Here's how the part is built. I have some questions about the finished solid (model axes, mm). Round coordinates to 2 decimals unless told otherwise and drop trailing zeros. Loops run counter-clockwise (first coordinate to the right, second up) from the corner with the lowest first, then second, coordinate; pieces in that order, holes last. Notation, with made-up numbers: M 81.5,-33 L 113.5,-33 A7 cw 113.5,-28 Z; hole C 42,62 d4. An arc over 180 degrees is marked long. Answer as a JSON object with one key per item and string values.
from build123d import *

# Parameters (mm, degrees)
BOSS_EXTRUDE1_DEPTH = 3
SKETCH3_W           = 102.374795857
SKETCH3_H           = 90.967021537
SKETCH3_W_2         = 153.648776174
SKETCH3_H_2         = 69.94350062
CUT_EXTRUDE2_DEPTH  = 10
CUT_EXTRUDE3_DEPTH  = 60


with BuildPart() as part:
    # Sketch1 → Boss-Extrude1 (new body)
    with BuildSketch(Plane(origin=(0, 0, 0), x_dir=(1, 0, 0), z_dir=(0, 1, 0))):
        Polygon((-245.183632637, 942.323086709), (-245.183632637, 742.323086709), (-145.183632637, 692.323086709), (126.532096115, 692.323086709), (154.816367363, 720.607357957), (154.816367363, 964.038815462), (126.532096115, 992.323086709), (-145.183632637, 992.323086709), align=None)
    extrude(amount=BOSS_EXTRUDE1_DEPTH)

    # Sketch3 → Cut-Extrude2 (cut)
    with BuildSketch(Plane(origin=(0, 3, 0), x_dir=(1, 0, 0), z_dir=(0, 1, 0))):
        with Locations((-196.371030566, 977.806597478)):
            Rectangle(SKETCH3_W, SKETCH3_H)
        with Locations((-222.008020724, 717.351336399)):
            Rectangle(SKETCH3_W_2, SKETCH3_H_2)
    extrude(amount=-CUT_EXTRUDE2_DEPTH, mode=Mode.SUBTRACT)

    # Sketch4 → Cut-Extrude3 (cut)
    with BuildSketch(Plane(origin=(0, 3, 0), x_dir=(1, 0, 0), z_dir=(0, 1, 0))):
        Polygon((-145.183632637, 947.323086709), (-100.183632637, 992.323086709), (-145.183632637, 992.323086709), align=None)
        Polygon((-100.183632637, 692.323086709), (-145.183632637, 692.323086709), (-145.183632637, 737.323086709), align=None)
    extrude(amount=-CUT_EXTRUDE3_DEPTH, mode=Mode.SUBTRACT)


solid = part.part
Item 1: I want a section at A-A, the plane y = 0.65. Please give me the cut outline in (x, z), then the cut area to 3 significant figures.
Resolved:
{"outline": "M -245.18,-932.32 L -145.18,-932.32 L -145.18,-947.32 L -100.18,-992.32 L 126.53,-992.32 L 154.82,-964.04 L 154.82,-720.61 L 126.53,-692.32 L -100.18,-692.32 L -145.18,-737.32 L -145.18,-752.32 L -245.18,-752.32 Z", "area": "105,000 mm²"}
Item 2: I'm going to push flat-ended pins straight in: pin 1 Ø0.9 at (y, z) = (1.5, -742) entering from -X; pin 2 Ø1.5 at (y, z) = (0.5, -735) entering from -X; pin 3 Ø0.9 at (x, y) = (-207.5, 2) entering from +Z. Where does each tip first touch, or does it pass through?
Resolved:
{"pin 1": "x = -145.18", "pin 2": "x = -143.61", "pin 3": "z = -752.32"}
Item 3: Please list where these lines run through material, in increasing order: probe 1 along X at (y, z) = (2.95, -945.5); probe 2 along X at (y, z) = (2.7, -732); probe 3 along Z at (x, y) = (-129.5, 0.2). Write a range as from..to.
Resolved:
{"probe 1": "-145.18..154.82", "probe 2": "-139.86..154.82", "probe 3": "-963.01..-721.64"}
Item 4: I want a section at B-B, the plane x = -113. Please give me the cut outline in (y, z), then the cut area to 3 significant figures.
Resolved:
{"outline": "M 0,-979.51 L 3,-979.51 L 3,-705.14 L 0,-705.14 Z", "area": "823 mm²"}
